Build history of the part. All positions in model axes, mm. A direction names the side the tool comes from. Give positions to 0.01 mm unless a question says otherwise; leave off trailing zeros. Order: outer loops, then holes, each group sorted by start corner. A loop starts at its lowest first (then second) coordinate and runs counter-clockwise, first axis right, second up. Notation, with made-up numbers: (66, 85.5) - (107, 85.5) arc R8 ccw to (107, 91.5) - close; hole circle Ø2 at (-18, 28). An arc over 180 degrees is marked (long way). Use a Markdown table: item, result. Add a question column.
(1) Slice it at C-C (y = 15). Count the separate pieces of the cut face and the enclosed holes in it, then the cut area to 3 significant figures.
(2) Slice it at A-A (x = 27.75). Write the cut outline in (y, z), then the cut area to 3 significant figures.
(3) Which spindle directions (+Z, -Z, +X, -X, +Y, -Y) get a long thin tool onto all of the face, cutting with end or side? Do faces 5 (the face through (40.252, 12.1, -91.2)), 6 (the face through (33.94, 15.91, -1.97)), 7 (the face through (46.26, 9.86, -5.2)). Say none if no direction does.
(4) Flat gauge pins, fed straight in: pin 1 (6 mm diameter, centred on x = 40, y = 15.5, fed in from -Z); pin 2 (2.5 mm diameter, centred on y = 10, z = -90, fed in from -X); pin 3 (6 mm diameter, centred on x = 29, y = 6, fed in from -Z); pin 4 (2 mm diameter, centred on x = 39, y = 2, fed in from -Z). Where does each tip first touch, or does it go through?
(5) Slice it at D-D (z = -49.5). Write the cut outline in (x, y), then the cut area to 3 significant figures.
(6) Mould opens along Y. For faces 1 (the face through (44.25, 14.93, -1.97)), 2 (the face through (27.577, 15.466, -91.426)), 3 (the face through (24.753, 10.132, -1.479)), 4 (the face through (15.252, 12, -58)) say: +Y half, -Y half, draft (parallel to the pull), parting line (faces both ways), or undercut.
(7) Wall check: line 1 (Y direction, x = 12.75, z = -2.4); line 2 (Y direction, x = 39, z = -84.5); line 3 (X direction, y = 13.5, z = -78.5). Give the ranges that are in metal, low to high.
(8) Slice it at B-B (x = 19.5). Write the cut outline in (y, z), then the cut area to 3 significant figures.
from build123d import *

# Parameters (mm, degrees)
EXTRUDE_1_DEPTH     = 20
SKETCH_2_R          = 1.5
CUT_EXTRUDE_1_DEPTH = 5
SKETCH_3_R          = 3
CUT_EXTRUDE_2_DEPTH = 3
SKETCH_4_W          = 24.99770673
SKETCH_4_H          = 59.73
CUT_EXTRUDE_3_DEPTH = 7
EXTRUDE_2_DEPTH     = 25
SKETCH_6_R          = 2.15
CUT_EXTRUDE_4_DEPTH = 104.292213424
FILLET_4_R          = 10
FILLET_5_R          = 10


with BuildPart() as part:
    # 스케치1 → 보스-돌출1 (new body)
    with BuildSketch(Plane(origin=(0, 0, 0), x_dir=(1, 0, 0), z_dir=(0, 1, 0))):
        Polygon((40.24770673, 90), (15.25229327, 90), (15.25229327, 17.25229327), (0, 2), (0, 0), (55.5, 0), (55.5, 2), (40.24770673, 17.25229327), align=None)
        with BuildLine():
            Line((11.071067812, 4), (44.428932188, 4))
            ThreePointArc((44.428932188, 4), (46.276691253, 5.234633135), (45.843145751, 7.414213562))
            Line((45.843145751, 7.414213562), (29.164213562, 24.093145751))
            ThreePointArc((29.164213562, 24.093145751), (27.75, 24.678932188), (26.335786438, 24.093145751))
            Line((26.335786438, 24.093145751), (9.656854249, 7.414213562))
            ThreePointArc((9.656854249, 7.414213562), (9.223308747, 5.234633135), (11.071067812, 4))
        make_face(mode=Mode.SUBTRACT)
    extrude(amount=EXTRUDE_1_DEPTH)

    # 스케치2 → 컷-돌출1 (cut)
    with BuildSketch(Plane.XY):
        with Locations((12.75, 15)):
            Circle(SKETCH_2_R)
        with Locations((22.75, 15)):
            Circle(SKETCH_2_R)
        with Locations(Location((32.75, 15, 0), (0, 0, 180))):
            Circle(SKETCH_2_R)
        with Locations(Location((42.75, 15, 0), (0, 0, 180))):
            Circle(SKETCH_2_R)
        with Locations((42.75, 5)):
            Circle(SKETCH_2_R)
        with Locations((32.75, 5)):
            Circle(SKETCH_2_R)
        with Locations(Location((22.75, 5, 0), (0, 0, 180))):
            Circle(SKETCH_2_R)
        with Locations(Location((12.75, 5, 0), (0, 0, 180))):
            Circle(SKETCH_2_R)
    extrude(amount=-CUT_EXTRUDE_1_DEPTH, mode=Mode.SUBTRACT)

    # 스케치3 → 컷-돌출2 (cut)
    with BuildSketch(Plane.XY):
        with Locations((27.75, 10)):
            Circle(SKETCH_3_R)
    extrude(amount=-CUT_EXTRUDE_2_DEPTH, mode=Mode.SUBTRACT)

    # 스케치4 → 컷-돌출3 (cut)
    with BuildSketch(Plane.XZ):
        with Locations((27.748853365, -60.135)):
            Rectangle(SKETCH_4_W, SKETCH_4_H)
    extrude(amount=-CUT_EXTRUDE_3_DEPTH, mode=Mode.SUBTRACT)

    # 스케치5 → 보스-돌출2 (add)
    with BuildSketch(Plane.ZY.offset(-15.25229327)):
        with BuildLine():
            Line((-90, 20), (-92.892384696, 10.804147089))
            ThreePointArc((-92.892384696, 10.804147089), (-92.390282771, 8.184258847), (-90, 7))
            Line((-90, 7), (-90, 20))
        make_face()
    extrude(amount=-EXTRUDE_2_DEPTH)

    # 스케치6 → 컷-돌출4 (cut, through all)
    with BuildSketch(Plane.ZY.offset(-15.25229327)):
        with Locations((-90.002169099, 9.999999216)):
            Circle(SKETCH_6_R)
    extrude(amount=-CUT_EXTRUDE_4_DEPTH, mode=Mode.SUBTRACT)

    # 필렛4
    fillet_4_edges = [part.edges().sort_by_distance(p)[0] for p in [
        (15.25229327, 10, -17.25229327),
        (40.24770673, 10, -17.25229327),
    ]]
    fillet(fillet_4_edges, radius=FILLET_4_R)

    # 필렛5
    # the kernel refuses this fillet: 10 mm, written as the material it adds along each edge
    with BuildSketch(Plane(origin=(15.25229327, 7, -30.27), x_dir=(0, -1, 0), z_dir=(1, 0, 0))) as fillet_5_piece_1:
        with BuildLine():
            CenterArc((10, 9.539392014), FILLET_5_R, 180, 72.542396876)
            Line((0, 9.539392014), (-0.2, 9.539392014))
            Line((-0.2, 9.539392014), (-0.2, 0))
            Line((-0.2, 0), (0, -0.2))
            ThreePointArc((0, -0.2), (3.5, -0.2), (6.94, -0.19078784))
            Line((6.94, -0.19078784), (7, 0))
        make_face()
    extrude(amount=24.99541346)


solid = part.part
Solution:
| question | item | result |
|---|---|---|
| 1 | separate pieces | 4 |
| 1 | enclosed holes | 0 |
| 1 | area | 2,090 mm2 |
| 2 | outline | (0, -30.27) arc R10 cw to (7, -39.81) - (7, -90) arc R3 ccw to (10.8, -92.89) - (20, -90) - (20, -24.68) - (0, -24.68) - close; (0, -4) - (20, -4) - (20, 0) - (13, 0) - (13, -3) - (7, -3) - (7, 0) - (0, 0) - close; hole circle Ø4.3 at (10, -90) |
| 2 | area | 976 mm2 |
| 3 | face 5 | -Z, +X, +Y, -Y |
| 3 | face 6 | +Z |
| 3 | face 7 | +Y, -Y |
| 4 | pin 1 | z = -92.36 |
| 4 | pin 2 | through |
| 4 | pin 3 | z = -92.83 |
| 4 | pin 4 | z = -31.81 |
| 5 | outline | (15.25, 7) - (40.25, 7) - (40.25, 20) - (15.25, 20) - close |
| 5 | area | 325 mm2 |
| 6 | face 1 | undercut |
| 6 | face 2 | +Y half |
| 6 | face 3 | undercut |
| 6 | face 4 | draft |
| 7 | line 1 | 0 to 3.5, 6.5 to 13.5, 16.5 to 20 |
| 7 | line 2 | 7 to 20 |
| 7 | line 3 | 15.25 to 40.25 |
| 8 | outline | (0, -30.27) arc R10 cw to (7, -39.81) - (7, -90) arc R3 ccw to (10.8, -92.89) - (20, -90) - (20, -17.26) - (0, -17.26) - close; (0, -4) - (20, -4) - (20, 0) - (0, 0) - close; hole circle Ø4.3 at (10, -90) |
| 8 | area | 1,140 mm2 |
